Verification items for the finished model (mm, model axes). Coordinates: 2 decimals unless noted, no trailing zeros. Order: outer loops, then holes, each group sorted by start corner. A loop starts at its lowest first (then second) coordinate and runs counter-clockwise, first axis right, second up. Notation, with made-up numbers: M 20,49 L 30,49 A19 ccw 30,58 Z; hole C -27,34.5 d2. An arc over 180 degrees is marked long. Answer as a JSON object with one key per item and string values. Group by question number.
(1) Cross-section at C-C (z = -0.25). Enter the section's corners in (x, y).
(2) Cross-section at B-B (x = 3.5). Enter the section's corners in (y, z).
(3) Gauge pin test, flat end, axial feed: pin 1 Ø3 at (x, y) = (2.5, -0.5) entering from +Z. Record the tip position at first contact, or that the pin passes through.
(4) Cross-section at A-A (y = 1.75). Enter the section's corners in (x, z), plus the area to 3 significant figures.
(5) Material ranges on line 1 (Y direction, x = 0, z = 0.25); line 2 (X direction, y = 0, z = -0.1); line 3 (Y direction, x = -1.25, z = 0.15), recorded low to high.
from build123d import *

# Parameters (mm, degrees)
BOSS_EXTRUDE1_DEPTH = 0.4
FILLET1_R           = 0.6


with BuildPart() as part:
    # Sketch1 → Boss-Extrude1 (new, symmetric)
    with BuildSketch(Plane.XY):
        with BuildLine():
            Line((-0.064573904, -3.699436472), (-0.08202631, -4.699284167))
            ThreePointArc((-0.08202631, -4.699284167), (-0.692406371, -5.28872134), (-0.102969198, -5.899101401))
            Line((-0.102969198, -5.899101401), (-0.120421604, -6.898949097))
            ThreePointArc((-0.120421604, -6.898949097), (-0.95172367, -6.834048731), (-1.769127189, -6.669346969))
            Line((-1.769127189, -6.669346969), (-2.471645104, -3.760448175))
            ThreePointArc((-2.471645104, -3.760448175), (0, 5.2), (2.471645104, -3.760448175))
            Line((2.471645104, -3.760448175), (1.769127189, -6.669346969))
            ThreePointArc((1.769127189, -6.669346969), (0.95172367, -6.834048731), (0.120421604, -6.898949097))
            Line((0.120421604, -6.898949097), (0.102969198, -5.899101401))
            ThreePointArc((0.102969198, -5.899101401), (0.692406371, -5.28872134), (0.08202631, -4.699284167))
            Line((0.08202631, -4.699284167), (0.064573904, -3.699436472))
            ThreePointArc((0.064573904, -3.699436472), (0, 3.7), (-0.064573904, -3.699436472))
        make_face()
    extrude(amount=BOSS_EXTRUDE1_DEPTH, both=True)

    # Fillet1
    fillet1_edges = [part.edges().sort_by_distance(p)[0] for p in [
        (-1.769127189, -6.669346969, 0),
        (-2.471645104, -3.760448175, 0),
        (2.471645104, -3.760448175, 0),
        (1.769127189, -6.669346969, 0),
    ]]
    fillet(fillet1_edges, radius=FILLET1_R)


solid = part.part
Taken from the geometry:
{
 "1": {"outline": "M -2.67,-3.64 A0.6 cw -2.41,-4 L -1.86,-6.31 A0.6 ccw -1.39,-6.76 A6.9 ccw -0.12,-6.9 L -0.1,-5.9 A0.6 cw -0.08,-4.7 L -0.06,-3.7 A3.7 cw long 0.06,-3.7 L 0.08,-4.7 A0.6 cw 0.1,-5.9 L 0.12,-6.9 A6.9 ccw 1.39,-6.76 A0.6 ccw 1.86,-6.31 L 2.41,-4 A0.6 cw 2.67,-3.64 A4.82 ccw long Z"},
 "2": {"outline": "M -2.94,-0.4 L -1.2,-0.4 L -1.2,0.4 L -2.94,0.4 Z; M 1.2,-0.4 L 3.69,-0.4 L 3.69,0.4 L 1.2,0.4 Z"},
 "3": {"pin 1": "stops at z = 0.4"},
 "4": {"outline": "M -4.62,-0.4 L -3.26,-0.4 L -3.26,0.4 L -4.62,0.4 Z; M 3.26,-0.4 L 4.62,-0.4 L 4.62,0.4 L 3.26,0.4 Z", "area": "2.18 mm²"},
 "5": {"line 1": "y = 3.7 to 5.2", "line 2": "x = -4.81 to -3.7, 3.7 to 4.81", "line 3": "y = -6.79 to -3.48, 3.48 to 5.04"}
}
